For this review, take the finished solid that the model builds, in its own axes (mm). A direction names the side the tool comes from. Round coordinates to 2 decimals unless told otherwise and drop trailing zeros. Loops run counter-clockwise (first coordinate to the right, second up) from the corner with the lowest first, then second, coordinate; pieces in that order, holes last. Notation, with made-up numbers: M 30,68.25 L 47,68.25 A23 cw 47,100.25 Z; hole C 24,12.25 d8. An arc over 180 degrees is marked long. One line per question, with ' | ' between items. Start each with the question number.
1) We need section D-D (x = 6.75). Give the boundary of the cut face in (y, z), and give its area (3 significant figures).
2) For faces 1 (the face through (-10.69, 4.64, 2.46)), 2 (the face through (7.06, -7.08, 2.46)), 3 (the face through (2.601, 9.656, 2.465)), 4 (the face through (9.415, -6.956, 2.465)), list the 3-axis set-ups (+Z, -Z, +X, -X, +Y, -Y) from which the entire face can be reached by the end or side of a thin tool; tool diameter is ignored.
3) We need section C-C (y = -11.5). Give the boundary of the cut face in (x, z), and give its area (3 significant figures).
4) We need section A-A (y = 0). Give the boundary of the cut face in (x, z), and give its area (4 significant figures).
5) We need section B-B (x = 0). Give the boundary of the cut face in (y, z).
6) Mouldability with a two-part tool opening along X and no side actions: class faces 5 (the face through (6.687, -11.554, 2.465)), 6 (the face through (-9.656, 2.601, 2.465)), 7 (the face through (2.58, -9.66, 2.46)) as pulls with the +X half, pulls with the -X half, needs draft (parallel to the pull), parting line crosses it, or undercut.
7) For probe 1 along Y at (x, z) = (0, 3.9); probe 2 along Y at (x, z) = (-11.5, 0.5); probe 3 along X at (y, z) = (0, 4), list the stretches that pass through material, from the lowest coordinate up. Write a range as from..to.
8) For pin 1 Ø3 at (x, z) = (7.5, 2.5) entering from -Y, flat-tipped, find the tip position at first contact; note if it passes through.
```python
from build123d import *

# Parameters (mm, degrees)
SKETCH1_R           = 10
BOSS_EXTRUDE1_DEPTH = 5
BOSS_EXTRUDE2_DEPTH = 5
CIRPATTERN1_COUNT   = 12
CUT_EXTRUDE1_DEPTH  = 7


with BuildPart() as part:
    # Sketch1 → Boss-Extrude1 (new body)
    with BuildSketch(Plane.XY):
        Circle(SKETCH1_R)
    extrude(amount=BOSS_EXTRUDE1_DEPTH)

    # Sketch3 → Boss-Extrude2 (add)
    with BuildSketch(Plane.XY):
        Polygon((-1, 13.35), (1, 13.35), (1.8, 9), (-1.8, 9), align=None)
    boss_extrude2 = extrude(amount=BOSS_EXTRUDE2_DEPTH)

    # CirPattern1: Boss-Extrude2 ×12 about axis
    cirpattern1_axis = Axis((0, 0, 0), (0, 0, 1))
    for i in range(1, CIRPATTERN1_COUNT):
        add(boss_extrude2.rotate(cirpattern1_axis, i * 360 / CIRPATTERN1_COUNT))

    # Sketch4 → Cut-Extrude1 (cut)
    with BuildSketch(Plane.XY):
        with BuildLine():
            Line((1.9, 3.405877273), (1.9, -3.405877273))
            ThreePointArc((1.9, -3.405877273), (-3.9, 0), (1.9, 3.405877273))
        make_face()
    extrude(amount=CUT_EXTRUDE1_DEPTH, mode=Mode.SUBTRACT)


solid = part.part
```
Answers below:
1) outline: M -11.52,0 L -8.84,0 L -8.84,5 L -11.52,5 Z; M -7.38,0 L 7.38,0 L 7.38,5 L -7.38,5 Z; M 8.84,0 L 11.52,0 L 11.52,5 L 8.84,5 Z | area: 101 mm^2
2) face 1: +Z, -Z, -X | face 2: +Z, -Z | face 3: +Z, -Z, +Y | face 4: +Z, -Z, -Y
3) outline: M -6.78,0 L -5.33,0 L -5.33,5 L -6.78,5 Z; M -1.34,0 L 1.34,0 L 1.34,5 L -1.34,5 Z; M 5.33,0 L 6.78,0 L 6.78,5 L 5.33,5 Z | area: 27.9 mm^2
4) outline: M -13.35,0 L -3.9,0 L -3.9,5 L -13.35,5 Z; M 1.9,0 L 13.35,0 L 13.35,5 L 1.9,5 Z | area: 104.5 mm^2
5) outline: M -13.35,0 L -3.9,0 L -3.9,5 L -13.35,5 Z; M 3.9,0 L 13.35,0 L 13.35,5 L 3.9,5 Z
6) face 5: pulls with the +X half | face 6: pulls with the -X half | face 7: undercut
7) probe 1: -13.35..-3.9, 3.9..13.35 | probe 2: -6.78..-5.33, -1.34..1.34, 5.33..6.78 | probe 3: -13.35..-3.9, 1.9..13.35
8) pin 1: y = -11.95
